Source: CAD feature listing. Evaluate the final solid. Frame: model axes, mm. Round coordinates to 2 decimals unless told otherwise and drop trailing zeros. Order: outer loops, then holes, each group sorted by start corner. A loop starts at its lowest first (then second) coordinate and runs counter-clockwise, first axis right, second up. Notation, with made-up numbers: (-5, 64.25) - (43, 64.25) arc R22 cw to (43, 70.25) - close; hole circle Ø11 at (40.5, 88). An arc over 180 degrees is marked (long way). Put each result on its own line as item: value. Start each with the question number.
1) Line query: probe 1 along Z at (x, y) = (-2, 16.25); probe 2 along Y at (x, z) = (23, -19.5); probe 3 along X at (y, z) = (1.5, 8.5). Output: solid intervals per line, ascending. Write a range as [from, to].
2) Contact query for flat-ended pins moving along their axis: P1, Ø1.5, axis at y = 8, z = -8.5, coming from the +X side; P2, Ø1, axis at x = -24.5, y = 12.5, coming from the +Z side; P3, Ø3, axis at x = 23, y = 4, coming from the +Z side. Output: stop coordinate, or through.
3) Section D-D on y = -2. Output: boundary loops of the cut face in (x, z).
4) Section A-A on x = 0. Output: boundary loops of the cut face in (y, z).
5) Section B-B on y = 9.5. State how many separate pieces and enclosed holes the cut face has, then the cut area to 3 significant figures.
6) Section C-C on z = -11. Output: boundary loops of the cut face in (x, y), then the cut area to 3 significant figures.
```python
from build123d import *

# Parameters (mm, degrees)
SKETCH1_R           = 39.5
BOSS_EXTRUDE1_DEPTH = 18
BOSS_EXTRUDE2_START = 5
SKETCH2_R           = 39.5
BOSS_EXTRUDE2_DEPTH = 5
SKETCH3_R           = 2.5
BOSS_EXTRUDE3_DEPTH = 20


with BuildPart() as part:
    # Sketch1 → Boss-Extrude1 (new body)
    with BuildSketch(Plane(origin=(0, 0, 0), x_dir=(1, 0, 0), z_dir=(0, 1, 0))):
        with Locations(Location((0, 0, 0), (0, 0, 270))):
            Circle(SKETCH1_R)
        with BuildLine():
            ThreePointArc((-5.301518913, 33.077846018), (-4.402379143, 33.209472412), (-3.5, 33.316662498))
            Line((-3.5, 33.316662498), (-1.5, 34.316662498))
            Line((-1.5, 34.316662498), (3.410400922, 34.316662498))
            Line((3.410400922, 34.316662498), (1.691602889, 33.457263481))
            ThreePointArc((1.691602889, 33.457263481), (2.598460964, 33.399071853), (3.50340703, 33.316304405))
            Line((3.50340703, 33.316304405), (5.667613922, 33.878628624))
            Line((5.667613922, 33.878628624), (10.470710803, 32.857698865))
            Line((10.470710803, 32.857698865), (8.610793528, 32.374437985))
            ThreePointArc((8.610793528, 32.374437985), (9.485735858, 32.128971587), (10.353698361, 31.85986394))
            Line((10.353698361, 31.85986394), (12.58752592, 31.959936111))
            Line((12.58752592, 31.959936111), (17.073400377, 29.962696124))
            Line((17.073400377, 29.962696124), (15.153651171, 29.876694198))
            ThreePointArc((15.153651171, 29.876694198), (15.958438578, 29.454681091), (16.751483392, 29.01099454))
            Line((16.751483392, 29.01099454), (18.957302633, 28.644441029))
            Line((18.957302633, 28.644441029), (22.929900428, 25.758179785))
            Line((22.929900428, 25.758179785), (21.034221542, 26.073195511))
            ThreePointArc((21.034221542, 26.073195511), (21.733680954, 25.493079692), (22.417148215, 24.894205468))
            Line((22.417148215, 24.894205468), (24.498554253, 24.077046424))
            Line((24.498554253, 24.077046424), (27.7842538, 20.427907387))
            Line((27.7842538, 20.427907387), (25.995495498, 21.130173066))
            ThreePointArc((25.995495498, 21.130173066), (26.559057183, 20.417308381), (27.103076093, 19.689420162))
            Line((27.103076093, 19.689420162), (28.969101496, 18.457369355))
            Line((28.969101496, 18.457369355), (31.424301957, 14.204837413))
            Line((31.424301957, 14.204837413), (29.820641561, 15.263660665))
            ThreePointArc((29.820641561, 15.263660665), (30.223675169, 14.449202721), (30.60446949, 13.624112715))
            Line((30.60446949, 13.624112715), (32.173559995, 12.031016677))
            Line((32.173559995, 12.031016677), (33.690957329, 7.360947882))
            Line((33.690957329, 7.360947882), (32.342482492, 8.73005305))
            ThreePointArc((32.342482492, 8.73005305), (32.567373521, 7.849597567), (32.768300713, 6.963366166))
            Line((32.768300713, 6.963366166), (33.971879535, 5.078850838))
            Line((33.971879535, 5.078850838), (34.485156198, 0.195349606))
            Line((34.485156198, 0.195349606), (33.450801742, 1.814900225))
            ThreePointArc((33.450801742, 1.814900225), (33.487698177, 0.907783468), (33.5, 0))
            ThreePointArc((33.5, 0), (33.499999989, -0.000856449), (33.499999956, -0.001712898))
            Line((33.499999956, -0.001712898), (34.285464925, -2.095285152))
            Line((34.285464925, -2.095285152), (33.772188263, -6.978786385))
            Line((33.772188263, -6.978786385), (33.097160441, -5.179572449))
            ThreePointArc((33.097160441, -5.179572449), (32.944495111, -6.075379978), (32.76758845, -6.966717101))
            Line((32.76758845, -6.966717101), (33.100610978, -9.177847128))
            Line((33.100610978, -9.177847128), (31.583213644, -13.847915922))
            Line((31.583213644, -13.847915922), (31.297014411, -11.947672952))
            ThreePointArc((31.297014411, -11.947672952), (30.961436327, -12.792164031), (30.603076093, -13.627242336))
            Line((30.603076093, -13.627242336), (30.469101496, -15.859293143))
            Line((30.469101496, -15.859293143), (28.013901035, -20.111825085))
            Line((28.013901035, -20.111825085), (28.129038671, -18.193602816))
            ThreePointArc((28.129038671, -18.193602816), (27.625214205, -18.949869132), (27.10106246, -19.69219169))
            Line((27.10106246, -19.69219169), (26.505946073, -21.847611947))
            Line((26.505946073, -21.847611947), (23.220246526, -25.496750984))
            Line((23.220246526, -25.496750984), (23.731688964, -23.644384934))
            ThreePointArc((23.731688964, -23.644384934), (23.081637663, -24.27937402), (22.414602352, -24.896497774))
            Line((22.414602352, -24.896497774), (21.384353616, -26.881085273))
            Line((21.384353616, -26.881085273), (17.41175582, -29.767346518))
            Line((17.41175582, -29.767346518), (18.297150571, -28.061793973))
            ThreePointArc((18.297150571, -28.061793973), (17.529282796, -28.547753758), (16.748516565, -29.012707438))
            Line((16.748516565, -29.012707438), (15.328162292, -30.739726182))
            Line((15.328162292, -30.739726182), (10.842287835, -32.736966169))
            Line((10.842287835, -32.736966169), (12.062938899, -31.252767959))
            ThreePointArc((12.062938899, -31.252767959), (11.210814157, -31.56845967), (10.350440235, -31.860922569))
            Line((10.350440235, -31.860922569), (8.602056724, -33.254893551))
            Line((8.602056724, -33.254893551), (3.798959843, -34.27582331))
            Line((3.798959843, -34.27582331), (5.301518913, -33.077846018))
            ThreePointArc((5.301518913, -33.077846018), (4.402379143, -33.209472412), (3.5, -33.316662498))
            Line((3.5, -33.316662498), (1.5, -34.316662498))
            Line((1.5, -34.316662498), (-3.410400922, -34.316662498))
            Line((-3.410400922, -34.316662498), (-1.691602889, -33.457263481))
            ThreePointArc((-1.691602889, -33.457263481), (-2.598460964, -33.399071853), (-3.50340703, -33.316304405))
            Line((-3.50340703, -33.316304405), (-5.667613922, -33.878628624))
            Line((-5.667613922, -33.878628624), (-10.470710803, -32.857698865))
            Line((-10.470710803, -32.857698865), (-8.610793528, -32.374437985))
            ThreePointArc((-8.610793528, -32.374437985), (-9.485735858, -32.128971587), (-10.353698361, -31.85986394))
            Line((-10.353698361, -31.85986394), (-12.587525919, -31.959936111))
            Line((-12.587525919, -31.959936111), (-17.073400377, -29.962696124))
            Line((-17.073400377, -29.962696124), (-15.153651171, -29.876694198))
            ThreePointArc((-15.153651171, -29.876694198), (-15.958438577, -29.454681091), (-16.751483392, -29.01099454))
            Line((-16.751483392, -29.01099454), (-18.957302633, -28.644441029))
            Line((-18.957302633, -28.644441029), (-22.929900428, -25.758179785))
            Line((-22.929900428, -25.758179785), (-21.034221542, -26.073195511))
            ThreePointArc((-21.034221542, -26.073195511), (-21.733680954, -25.493079692), (-22.417148215, -24.894205468))
            Line((-22.417148215, -24.894205468), (-24.498554253, -24.077046424))
            Line((-24.498554253, -24.077046424), (-27.7842538, -20.427907387))
            Line((-27.7842538, -20.427907387), (-25.995495498, -21.130173066))
            ThreePointArc((-25.995495498, -21.130173066), (-26.559057183, -20.417308381), (-27.103076092, -19.689420162))
            Line((-27.103076092, -19.689420162), (-28.969101496, -18.457369355))
            Line((-28.969101496, -18.457369355), (-31.424301957, -14.204837413))
            Line((-31.424301957, -14.204837413), (-29.820641561, -15.263660665))
            ThreePointArc((-29.820641561, -15.263660665), (-30.223675169, -14.449202721), (-30.60446949, -13.624112715))
            Line((-30.60446949, -13.624112715), (-32.173559995, -12.031016677))
            Line((-32.173559995, -12.031016677), (-33.690957329, -7.360947882))
            Line((-33.690957329, -7.360947882), (-32.342482492, -8.73005305))
            ThreePointArc((-32.342482492, -8.73005305), (-32.567373521, -7.849597567), (-32.768300713, -6.963366166))
            Line((-32.768300713, -6.963366166), (-33.971879535, -5.078850838))
            Line((-33.971879535, -5.078850838), (-34.485156198, -0.195349606))
            Line((-34.485156198, -0.195349606), (-33.450801742, -1.814900225))
            ThreePointArc((-33.450801742, -1.814900225), (-33.487721374, -0.906927333), (-33.499999956, 0.001712898))
            Line((-33.499999956, 0.001712898), (-34.285464925, 2.095285152))
            Line((-34.285464925, 2.095285152), (-33.772188263, 6.978786385))
            Line((-33.772188263, 6.978786385), (-33.097160441, 5.179572449))
            ThreePointArc((-33.097160441, 5.179572449), (-32.944495111, 6.075379978), (-32.76758845, 6.966717101))
            Line((-32.76758845, 6.966717101), (-33.100610978, 9.177847128))
            Line((-33.100610978, 9.177847128), (-31.583213644, 13.847915922))
            Line((-31.583213644, 13.847915922), (-31.297014411, 11.947672952))
            ThreePointArc((-31.297014411, 11.947672952), (-30.961436327, 12.792164031), (-30.603076093, 13.627242336))
            Line((-30.603076092, 13.627242336), (-30.469101496, 15.859293143))
            Line((-30.469101496, 15.859293143), (-28.013901035, 20.111825085))
            Line((-28.013901035, 20.111825085), (-28.129038671, 18.193602816))
            ThreePointArc((-28.129038671, 18.193602816), (-27.625214205, 18.949869132), (-27.10106246, 19.69219169))
            Line((-27.10106246, 19.69219169), (-26.505946073, 21.847611947))
            Line((-26.505946073, 21.847611947), (-23.220246526, 25.496750984))
            Line((-23.220246526, 25.496750984), (-23.731688964, 23.644384934))
            ThreePointArc((-23.731688964, 23.644384934), (-23.081637663, 24.27937402), (-22.414602352, 24.896497774))
            Line((-22.414602352, 24.896497774), (-21.384353616, 26.881085273))
            Line((-21.384353616, 26.881085273), (-17.41175582, 29.767346518))
            Line((-17.41175582, 29.767346518), (-18.297150571, 28.061793973))
            ThreePointArc((-18.297150571, 28.061793973), (-17.529282796, 28.547753758), (-16.748516565, 29.012707438))
            Line((-16.748516565, 29.012707438), (-15.328162292, 30.739726182))
            Line((-15.328162292, 30.739726182), (-10.842287835, 32.736966169))
            Line((-10.842287835, 32.736966169), (-12.062938899, 31.252767959))
            ThreePointArc((-12.062938899, 31.252767959), (-11.210814157, 31.56845967), (-10.350440235, 31.860922569))
            Line((-10.350440235, 31.860922569), (-8.602056724, 33.254893551))
            Line((-8.602056724, 33.254893551), (-3.798959843, 34.27582331))
            Line((-3.798959843, 34.27582331), (-5.301518913, 33.077846018))
        make_face(mode=Mode.SUBTRACT)
    extrude(amount=BOSS_EXTRUDE1_DEPTH)

    # Sketch2 → Boss-Extrude2 (add)
    with BuildSketch(Plane(origin=(0, 0, 0), x_dir=(-1, 0, 0), z_dir=(0, -1, 0)).offset(BOSS_EXTRUDE2_START)):
        with Locations(Location((0, 0, 0), (0, 0, 90))):
            Circle(SKETCH2_R)
    extrude(amount=-BOSS_EXTRUDE2_DEPTH)

    # Sketch3 → Boss-Extrude3 (add)
    with BuildSketch(Plane(origin=(0, 0, 0), x_dir=(1, 0, 0), z_dir=(0, 1, 0))):
        with Locations(Location((0, 0, 0), (0, 0, 90))):
            Circle(SKETCH3_R)
    extrude(amount=BOSS_EXTRUDE3_DEPTH)


solid = part.part
```
Answer sheet:
1. probe 1: [-39.45, -34.07], [-1.5, 1.5], [33.44, 33.61], [34.32, 39.45]
1. probe 2: [-5, 0]
1. probe 3: [-38.57, -33.32], [-32.57, -32.4], [33, 38.57]
2. P1: x = 38.73
2. P2: z = 31.37
2. P3: z = 33.14
3. outline: circle Ø79 at (0, 0)
4. outline: (-5, -39.5) - (18, -39.5) - (18, -34.32) - (0, -34.32) - (0, -2.5) - (20, -2.5) - (20, 2.5) - (0, 2.5) - (0, 34.32) - (18, 34.32) - (18, 39.5) - (-5, 39.5) - close
5. separate pieces: 2
5. enclosed holes: 1
5. area: 1,270 mm^2
6. outline: (-37.94, -5) - (37.94, -5) - (37.94, 18) - (32.51, 18) - (32.51, 0) - (-32.51, 0) - (-32.51, 18) - (-37.94, 18) - close
6. area: 575 mm^2
